Here's the drawing with two shaded views (mm, measured from the low corner). I have some questions. A direction names the side the tool comes from. Give positions to 0.01 mm unless a question says otherwise; leave off trailing zeros. Order: outer loops, then holes, each group sorted by start corner. A loop starts at its lowest first (then second) coordinate and runs counter-clockwise, first axis right, second up. Notation, with made-up numbers: M -27,17 L 12,17 A36 cw 12,56 Z; hole C 75.25,-12 d2. An arc over 180 degrees is marked long. Write each question's results on one line, items separated by ' | '.
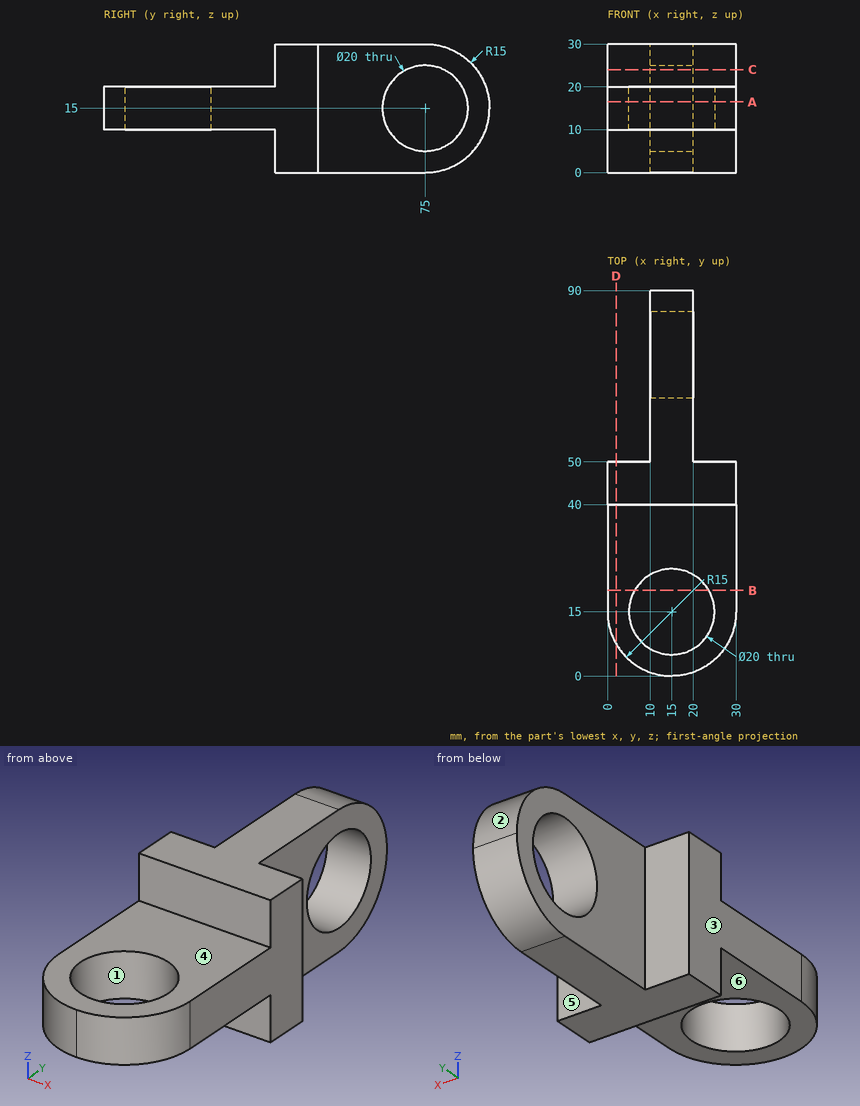
(1) Will these pins go through, and if not, where does the flat tip stop? P1, Ø15, axis at y = 78.5, z = 17, coming from the +X side; P2, Ø12, axis at x = 19, z = 11.5, coming from the +Y side; P3, Ø6, axis at x = 5, z = 21.5, coming from the +Y side; P4, Ø15, axis at y = 72, z = 18.5, coming from the -X side.
Data:
P1: stops at x = 20 | P2: stops at y = 90 | P3: stops at y = 50 | P4: stops at x = 10
(2) Imagine slicing it at B-B, the plane y = 20. Write out the boundary of the cut face in (x, z).
Data:
outline: M 0,10 L 6.34,10 L 6.34,20 L 0,20 Z; M 23.66,10 L 30,10 L 30,20 L 23.66,20 Z
(3) Imagine slicing it at A-A, the plane z = 16.5. Count the separate pieces of the cut face and the enclosed holes in it, plus the area to 3 significant figures.
Data:
separate pieces: 2 | enclosed holes: 1 | area: 1,290 mm2
(4) Imagine slicing it at C-C, the plane z = 24. Write out the boundary of the cut face in (x, y).
Data:
outline: M 0,40 L 30,40 L 30,50 L 20,50 L 20,70.64 L 10,70.64 L 10,50 L 0,50 Z; M 10,79.36 L 20,79.36 L 20,87 L 10,87 Z
(5) I need wall thicknesses on L1, parallel to Y at x = 15, z = 15.5; L2, parallel to Y at x = 15, z = 16.25; L3, parallel to Z at x = 13.25, y = 75. Which ranges of each line are inside material? Lowest first, please. Write a range as from..to.
Data:
L1: y = 0..5, 25..65.01, 84.99..89.99 | L2: y = 0..5, 25..65.08, 84.92..89.95 | L3: z = 0..5, 25..30
(6) For the marked faces 4, 5 and 6, which set-ups out of +Z, -Z, +X, -X, +Y, -Y let a thin tool reach every point of the face, with its end or its side?
Data:
face 4: +Z, +X, -X, -Y | face 5: +Z, -Z, +X, +Y | face 6: -Z, +X, -X, -Y
(7) Imagine slicing it at D-D, the plane x = 2. Write out the boundary of the cut face in (y, z), plus the area to 3 significant figures.
Data:
outline: M 7.52,10 L 40,10 L 40,0 L 50,0 L 50,30 L 40,30 L 40,20 L 7.52,20 Z | area: 625 mm2
(8) We'd pull the mould along Y, two halves only. Please class the marked faces 1, 2 and 3: +Y half, -Y half, draft (parallel to the pull), parting line (faces both ways), or undercut.
Data:
face 1: undercut | face 2: +Y half | face 3: draft
